Read the model definition and answer for the solid it produces. Units are mm, in the model's axes. Face numbers are marked on the shaded views. A direction names the side the tool comes from. Coordinates: 2 decimals unless noted, no trailing zeros. Write each loop counter-clockwise with the first axis right and the second up, starting at its lowest first coordinate (ties: lowest second). Pieces come first, ordered by that corner, then holes. Notation, with made-up numbers: (5, 82) -> (47, 82) arc R26 ccw to (47, 101) -> close; hole circle Ø9 at (34, 88). An arc over 180 degrees is marked (long way). One line per item, written item: value. Start each with the question number.
1. Find section C-C, the plane z = 2. Write down the section's boundary in (x, y), and give its area (3 significant figures).
2. For a pull along Y with two mould halves and no side action, classify the marked faces 1, 2 and 3 as pulls with the +Y half, pulls with the -Y half, needs draft (parallel to the pull), parting line crosses it, or undercut.
3. For the marked faces 4 and 5, determine the directions among +Z, -Z, +X, -X, +Y, -Y from which every point of the face is accessible in a straight line to the end or side of a thin tool.
4. Find section A-A, the plane x = 0. State how many separate pieces and enclosed holes the cut face has, and give its area (3 significant figures).
5. Given P1, Ø2.5, axis at y = 6, z = 10.5, coming from the -X side; P2, Ø5, axis at x = 0, z = 10.5, coming from the -Y side; P3, Ø3, axis at x = 1.5, z = 10, coming from the +Y side, each flat-ended and moving along its own axis, determine where each tip first touches the part or whether it passes through.
6. Find section B-B, the plane y = 0. Write down the section's boundary in (x, z), and give its area (3 significant figures).
7. Find section D-D, the plane z = 6.75. Write down the section's boundary in (x, y), and give its area (3 significant figures).
8. Consider line 1 along Y through (x, z) = (0, 7); line 2 along X through (y, z) = (-5, 1.5); line 3 along Y through (x, z) = (0, 3.75). Determine where each line is inside the solid, lowest interval first.
```python
from build123d import *

# Parameters (mm, degrees)
SKETCH_R             = 20
PAD_DEPTH            = 4
SKETCH001_R          = 1.6
POCKET_DEPTH         = 117.420575
POLARPATTERN_COUNT   = 5
SKETCH002_R          = 9
PAD001_DEPTH         = 10
SKETCH003_R          = 2.5
POCKET001_DEPTH      = 14.001
SKETCH004_W          = 5.8
SKETCH004_H          = 3
POCKET002_DEPTH      = 6.5
SKETCH005_R          = 1.6
POCKET003_DEPTH      = 6
POCKET003_DEPTH_BACK = -6
FILLET_R             = 1


with BuildPart() as part:
    # Sketch → Pad (new body)
    with BuildSketch(Plane.XY):
        Circle(SKETCH_R)
    extrude(amount=PAD_DEPTH)

    # Sketch001 (on Face3 of Pad) → Pocket (cut, through all)
    with BuildSketch(Plane.XY.offset(4)):
        with Locations((0, -13.3)):
            Circle(SKETCH001_R)
    pocket = extrude(amount=-POCKET_DEPTH, mode=Mode.SUBTRACT)

    # PolarPattern: Pocket ×5 about axis
    polarpattern_axis = Axis((0, 0, 4), (0, 0, 1))
    for i in range(1, POLARPATTERN_COUNT):
        add(pocket.rotate(polarpattern_axis, i * 360 / POLARPATTERN_COUNT), mode=Mode.SUBTRACT)

    # Sketch002 (on Face3 of PolarPattern) → Pad001 (join)
    with BuildSketch(Plane.XY.offset(4)):
        Circle(SKETCH002_R)
    extrude(amount=PAD001_DEPTH)

    # Sketch003 (on Face10 of Pad001) → Pocket001 (cut, through all)
    with BuildSketch(Plane.XY.offset(14)):
        Circle(SKETCH003_R)
    extrude(amount=-POCKET001_DEPTH, mode=Mode.SUBTRACT)

    # Sketch004 (on Face11 of Pocket001) → Pocket002 (cut)
    with BuildSketch(Plane.XY.offset(14)):
        with Locations((0, 5.5)):
            Rectangle(SKETCH004_W, SKETCH004_H)
    extrude(amount=-POCKET002_DEPTH, mode=Mode.SUBTRACT)

    # Sketch005 (on Face15 of Pocket002) → Pocket003 (cut, two sides)
    with BuildSketch(Plane.XZ.offset(-7)) as pocket003_sk:
        with Locations((0, 10.5)):
            Circle(SKETCH005_R)
    extrude(amount=-POCKET003_DEPTH, mode=Mode.SUBTRACT)
    extrude(pocket003_sk.sketch, amount=-POCKET003_DEPTH_BACK, mode=Mode.SUBTRACT)

    # Fillet
    fillet_edges = [part.edges().sort_by_distance(p)[0] for p in [
        (-20, 0, 4),
        (-9, 0, 14),
    ]]
    fillet(fillet_edges, radius=FILLET_R)


solid = part.part
```
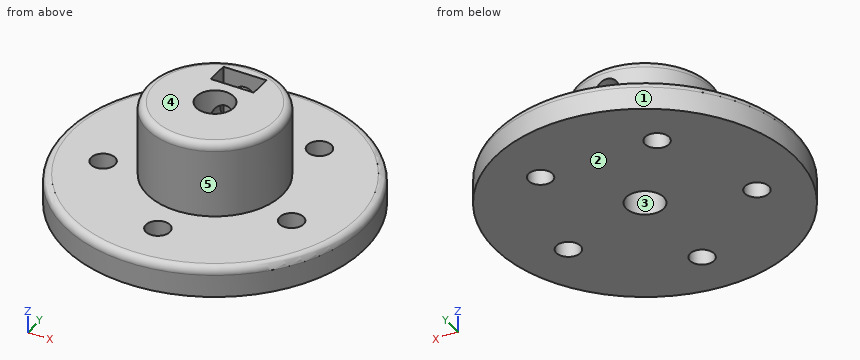
Answer block:
1. outline: circle Ø40 at (0, 0); hole circle Ø3.2 at (-12.65, -4.11); hole circle Ø3.2 at (-7.82, 10.76); hole circle Ø5 at (0, 0); hole circle Ø3.2 at (0, -13.3); hole circle Ø3.2 at (7.82, 10.76); hole circle Ø3.2 at (12.65, -4.11)
1. area: 1,200 mm2
2. face 1: parting line crosses it
2. face 2: needs draft
2. face 3: undercut
3. face 4: +Z, +X, -X, +Y, -Y
3. face 5: +Z
4. separate pieces: 5
4. enclosed holes: 0
4. area: 226 mm2
5. P1: stops at x = -7.64
5. P2: stops at y = -9
5. P3: stops at y = 8.99
6. outline: (-20, 0) -> (-2.5, 0) -> (-2.5, 14) -> (-8, 14) arc R1 ccw to (-9, 13) -> (-9, 4) -> (-19, 4) arc R1 ccw to (-20, 3) -> close; (2.5, 0) -> (20, 0) -> (20, 3) arc R1 ccw to (19, 4) -> (9, 4) -> (9, 13) arc R1 ccw to (8, 14) -> (2.5, 14) -> close
6. area: 269 mm2
7. outline: circle Ø18 at (0, 0); hole circle Ø5 at (0, 0)
7. area: 235 mm2
8. line 1: y = -9 to -2.5, 2.5 to 9
8. line 2: x = -19.36 to -13.98, -11.32 to 11.32, 13.98 to 19.36
8. line 3: y = -19.66 to -14.9, -11.7 to -2.5, 2.5 to 19.66
